```python
from build123d import *

# Parameters (mm, degrees)
SKETCH2_W           = 156
SKETCH2_H           = 48
SKETCH2_R           = 2.05
SKETCH2_R_2         = 7.05
BOSS_EXTRUDE2_DEPTH = 3.175
FILLET1_R           = 8
FILLET2_R           = 1


with BuildPart() as part:
    # Sketch2 → Boss-Extrude2 (new body)
    with BuildSketch(Plane.XY):
        Rectangle(SKETCH2_W, SKETCH2_H)
        with Locations((-70, 8)):
            Circle(SKETCH2_R, mode=Mode.SUBTRACT)
        with Locations((-54, 8)):
            Circle(SKETCH2_R, mode=Mode.SUBTRACT)
        with Locations((-54, -8)):
            Circle(SKETCH2_R, mode=Mode.SUBTRACT)
        with Locations((-70, -8)):
            Circle(SKETCH2_R, mode=Mode.SUBTRACT)
        with Locations((-39.5, 16)):
            Circle(SKETCH2_R, mode=Mode.SUBTRACT)
        with Locations((-39.5, -16)):
            Circle(SKETCH2_R, mode=Mode.SUBTRACT)
        with Locations((47.795580316, 0)):
            Circle(SKETCH2_R_2, mode=Mode.SUBTRACT)
        with Locations((-62, 0)):
            Circle(SKETCH2_R_2, mode=Mode.SUBTRACT)
        with Locations((72, 18)):
            Circle(SKETCH2_R, mode=Mode.SUBTRACT)
        with Locations((72, -18)):
            Circle(SKETCH2_R, mode=Mode.SUBTRACT)
        with Locations((-72, -18)):
            Circle(SKETCH2_R, mode=Mode.SUBTRACT)
        with Locations((-72, 18)):
            Circle(SKETCH2_R, mode=Mode.SUBTRACT)
        Polygon((7.35, -12), (-36.35, -12), (-36.35, -8), (-42, -8), (-42, 8), (-36.35, 8), (-36.35, 12), (7.35, 12), (7.35, 8), (13, 8), (13, -8), (7.35, -8), align=None, mode=Mode.SUBTRACT)
        with BuildLine():
            Line((10.5, 18.05), (13.5, 18.05))
            ThreePointArc((13.5, 18.05), (15.55, 16), (13.5, 13.95))
            Line((13.5, 13.95), (10.5, 13.95))
            ThreePointArc((10.5, 13.95), (8.45, 16), (10.5, 18.05))
        make_face(mode=Mode.SUBTRACT)
        with BuildLine():
            Line((-21.5, 13.95), (-18.5, 13.95))
            ThreePointArc((-18.5, 13.95), (-16.45, 16), (-18.5, 18.05))
            Line((-18.5, 18.05), (-21.5, 18.05))
            ThreePointArc((-21.5, 18.05), (-23.55, 16), (-21.5, 13.95))
        make_face(mode=Mode.SUBTRACT)
        with BuildLine():
            Line((-21.5, -18.05), (-18.5, -18.05))
            ThreePointArc((-18.5, -18.05), (-16.45, -16), (-18.5, -13.95))
            Line((-18.5, -13.95), (-21.5, -13.95))
            ThreePointArc((-21.5, -13.95), (-23.55, -16), (-21.5, -18.05))
        make_face(mode=Mode.SUBTRACT)
        with BuildLine():
            Line((10.5, -18.05), (13.5, -18.05))
            ThreePointArc((13.5, -18.05), (15.55, -16), (13.5, -13.95))
            Line((13.5, -13.95), (10.5, -13.95))
            ThreePointArc((10.5, -13.95), (8.45, -16), (10.5, -18.05))
        make_face(mode=Mode.SUBTRACT)
    extrude(amount=BOSS_EXTRUDE2_DEPTH)

    # Fillet1
    fillet1_edges = [part.edges().sort_by_distance(p)[0] for p in [
        (78, 24, 1.5875),
        (78, -24, 1.5875),
        (-78, -24, 1.5875),
        (-78, 24, 1.5875),
    ]]
    fillet(fillet1_edges, radius=FILLET1_R)

    # Fillet2
    fillet2_edges = [part.edges().sort_by_distance(p)[0] for p in [
        (7.35, 12, 1.5875),
        (-36.35, 12, 1.5875),
        (-36.35, 8, 1.5875),
        (-42, 8, 1.5875),
        (-42, -8, 1.5875),
        (-36.35, -8, 1.5875),
        (-36.35, -12, 1.5875),
        (7.35, -12, 1.5875),
        (7.35, -8, 1.5875),
        (13, -8, 1.5875),
        (13, 8, 1.5875),
        (7.35, 8, 1.5875),
    ]]
    fillet(fillet2_edges, radius=FILLET2_R)


solid = part.part
```
The model under review builds one solid part; all positions refer to its coordinate system, in mm. A direction names the side the tool comes from. Coordinates: 2 decimals unless noted, no trailing zeros. Order: outer loops, then holes, each group sorted by start corner. A loop starts at its lowest first (then second) coordinate and runs counter-clockwise, first axis right, second up. Notation, with made-up numbers: (72.5, 59.5) -> (119.5, 59.5) arc R19 cw to (119.5, 76.5) -> close; hole circle Ø4 at (-23.5, 25). An arc over 180 degrees is marked (long way). Answer in a Markdown table with one row per item. Add a question column.
Item 1: We need section A-A on x = -32. Write out the cut boundary in (y, z) (3 decimals).
Item 2: Clearance check with a flat-ended pin moving along its axis: pin 1 (3.5 mm diameter, centred on x = 72, y = 18, fed in from +Z). State where the tip first meets the part, or that it passes through.
Item 3: We need section C-C on x = -61.5. Write out the cut boundary in (y, z) (3 decimals), plus the area to 3 significant figures.
Item 4: We need section B-B on y = 2. Write out the cut boundary in (x, z) (3 decimals), plus the area to 3 significant figures.
Item 5: To check wall thickness, follow probe 1 along Y at (x, z) = (-39.5, 2.4); probe 2 along Y at (x, z) = (-54, 1.9); probe 3 along X at (y, z) = (-9, 2.4). State the ranges of each line that lie inside material, in increasing order.
Item 6: Machinability: for faces 1 (the flat face through (16, 0, 3.175)), 2 (the cylindrical face through (15.55, -16.05, 1.57)), which of the approach directions +Z, -Z, +X, -X, +Y, -Y give a long, thin tool a straight path to every point of the face, cutting with its end or side? Answer none if there is none.
Item 7: Mouldability with a two-part tool opening along X and no side actions: class faces 3 (the cylindrical face through (-74.05, 18.09, 1.57)), 4 (the cylindrical face through (-75.719, 21.594, 1.61)), 5 (the cylindrical face through (-56.05, -7.91, 1.57)), 6 (the cylindrical face through (75.594, 21.719, 1.61)) as +X half, -X half, draft (parallel to the pull), parting line (faces both ways), or undercut.
Final values:
| question | item | result |
|---|---|---|
| 1 | outline | (-24, 0) -> (-12, 0) -> (-12, 3.175) -> (-24, 3.175) -> close; (12, 0) -> (24, 0) -> (24, 3.175) -> (12, 3.175) -> close |
| 2 | pin 1 | passes through |
| 3 | outline | (-24, 0) -> (-7.032, 0) -> (-7.032, 3.175) -> (-24, 3.175) -> close; (7.032, 0) -> (24, 0) -> (24, 3.175) -> (7.032, 3.175) -> close |
| 3 | area | 108 mm2 |
| 4 | outline | (-78, 0) -> (-68.76, 0) -> (-68.76, 3.175) -> (-78, 3.175) -> close; (-55.24, 0) -> (-42, 0) -> (-42, 3.175) -> (-55.24, 3.175) -> close; (13, 0) -> (41.035, 0) -> (41.035, 3.175) -> (13, 3.175) -> close; (54.556, 0) -> (78, 0) -> (78, 3.175) -> (54.556, 3.175) -> close |
| 4 | area | 235 mm2 |
| 5 | probe 1 | y = -24 to -18.05, -13.95 to -8, 8 to 13.95, 18.05 to 24 |
| 5 | probe 2 | y = -24 to -10.05, -5.95 to 5.95, 10.05 to 24 |
| 5 | probe 3 | x = -78 to -71.79, -68.21 to -55.79, -52.21 to -36.35, 7.35 to 78 |
| 6 | face 1 | +Z, +X, -X, +Y, -Y |
| 6 | face 2 | +Z, -Z |
| 7 | face 3 | undercut |
| 7 | face 4 | -X half |
| 7 | face 5 | undercut |
| 7 | face 6 | +X half |
